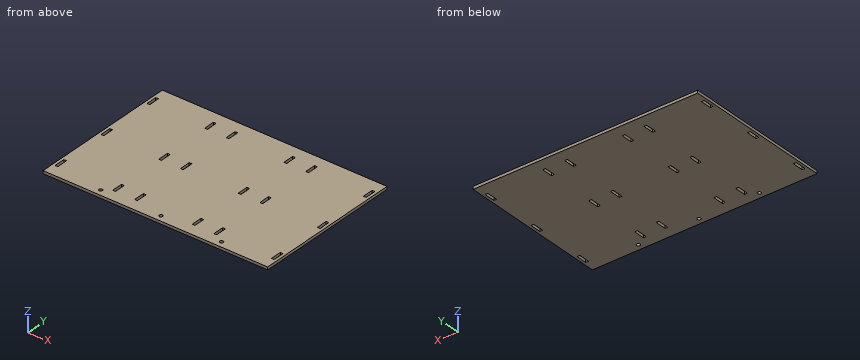
```python
from build123d import *

# Parameters (mm, degrees)
F0_W     = 6.35
F0_H     = 25.4
F0_R     = 3.96875
F1_DEPTH = 6.35


with BuildPart() as f1:
    # F0 (on Top) → F1 (new body)
    with BuildSketch(Plane.XY):
        Polygon((254, 146.3802), (254, 173.5), (-254, 173.5), (-260.35, 173.5), (-260.35, -173.5), (-254, -173.5), (254, -173.5), (254, -146.3802), (247.65, -146.3802), (247.65, -120.9802), (254, -120.9802), (254, -12.7), (247.65, -12.7), (247.65, 12.7), (254, 12.7), (254, 120.9802), (247.65, 120.9802), (247.65, 146.3802), align=None)
        with Locations((-250.825, -133.6802)):
            Rectangle(F0_W, F0_H, mode=Mode.SUBTRACT)
        with Locations((-138.1125, -159.2125)):
            Circle(F0_R, mode=Mode.SUBTRACT)
        with Locations((-117.175, -133.6802)):
            Rectangle(F0_W, F0_H, mode=Mode.SUBTRACT)
        with Locations((-66.825, -133.2992)):
            Rectangle(F0_W, F0_H, mode=Mode.SUBTRACT)
        with Locations((-250.825, 0)):
            Rectangle(F0_W, F0_H, mode=Mode.SUBTRACT)
        with Locations((-117.175, 0)):
            Rectangle(F0_W, F0_H, mode=Mode.SUBTRACT)
        with Locations((-66.825, 0)):
            Rectangle(F0_W, F0_H, mode=Mode.SUBTRACT)
        with Locations((1.5875, -159.2125)):
            Circle(F0_R, mode=Mode.SUBTRACT)
        with Locations((66.825, -133.2992)):
            Rectangle(F0_W, F0_H, mode=Mode.SUBTRACT)
        with Locations((117.175, -133.6802)):
            Rectangle(F0_W, F0_H, mode=Mode.SUBTRACT)
        with Locations((142.24, -159.2125)):
            Circle(F0_R, mode=Mode.SUBTRACT)
        with Locations((66.825, 0)):
            Rectangle(F0_W, F0_H, mode=Mode.SUBTRACT)
        with Locations((117.175, 0)):
            Rectangle(F0_W, F0_H, mode=Mode.SUBTRACT)
        with Locations((-250.825, 133.6802)):
            Rectangle(F0_W, F0_H, mode=Mode.SUBTRACT)
        with Locations((-117.175, 133.6802)):
            Rectangle(F0_W, F0_H, mode=Mode.SUBTRACT)
        with Locations((-66.825, 133.2992)):
            Rectangle(F0_W, F0_H, mode=Mode.SUBTRACT)
        with Locations((66.825, 133.2992)):
            Rectangle(F0_W, F0_H, mode=Mode.SUBTRACT)
        with Locations((117.175, 133.6802)):
            Rectangle(F0_W, F0_H, mode=Mode.SUBTRACT)
        Polygon((260.35, 173.5), (254, 173.5), (254, 146.3802), (254, 120.9802), (254, 12.7), (254, -12.7), (254, -120.9802), (254, -146.3802), (254, -173.5), (260.35, -173.5), align=None)
    extrude(amount=F1_DEPTH)


solid = f1.part
```
CAD build for the part. Positions are in the model's coordinates, mm. Coordinates: 2 decimals unless noted, no trailing zeros.
(1) Cut at A-A, the plane z = 4.25. Count the separate pieces of the cut face and the enclosed holes in it, and give its area (3 significant figures).
(2) Flat gauge pin, fed straight in: pin 1 (6.5 mm diameter, centred on x = 142.24, y = -159.21, fed in from -Z). Where does the tip first touch, or does it go through?
(3) Drill centre lines: probe 1 along Y at (x, z) = (-69.5, 4.5); probe 2 along Y at (x, z) = (142.24, 2.75). Where is each one in solid material? Low to high.
Geometry says:
1. separate pieces: 1
1. enclosed holes: 21
1. area: 178,000 mm2
2. pin 1: passes through
3. probe 1: y = -173.5 to -146, -120.6 to -12.7, 12.7 to 120.6, 146 to 173.5
3. probe 2: y = -173.5 to -163.18, -155.24 to 173.5
